from build123d import *

# Parameters (mm, degrees)
F0_R     = 3.175
F1_DEPTH = 3.048


with BuildPart() as f1:
    # F0 (on Front) → F1 (new body)
    with BuildSketch(Plane.XZ):
        with BuildLine():
            ThreePointArc((-23.2488528316, 63.9433400749), (-23.2457905964, 64.0827574545), (-23.2447697784, 64.222204724))
            ThreePointArc((-23.2447697784, 64.222204724), (-32.6010796562, 73.7457108348), (-42.2887946902, 64.5595320539))
            ThreePointArc((-42.2887946902, 64.5595320539), (-33.0778672203, 54.7021889169), (-23.2488528316, 63.9433400749))
        make_face()
        with Locations((-32.7697697784, 64.222204724)):
            Circle(F0_R, mode=Mode.SUBTRACT)
        with BuildLine():
            ThreePointArc((-23.2488528316, 63.9433400749), (-33.0778672203, 54.7021889169), (-42.2887946902, 64.5595320539))
            Line((-42.2887946902, 64.5595320539), (-48.5187123814, 15.4188098138))
            ThreePointArc((-48.5187123814, 15.4188098138), (-32.7820421912, 29.2971999803), (-17.023933011, 15.4431573445))
            Line((-17.023933011, 15.4431573445), (-23.2488528316, 63.9433400749))
        make_face()
        with Locations((-37.0385125279, 49.947404724)):
            Circle(F0_R, mode=Mode.SUBTRACT)
        with BuildLine():
            Line((-47.8670611639, 8.5143113042), (-48.5187123814, 15.4188098138))
            ThreePointArc((-48.5187123814, 15.4188098138), (-48.5745337038, 11.9305404647), (-47.8670611639, 8.5143113042))
        make_face()
        with BuildLine():
            ThreePointArc((-17.023933011, 15.4431573445), (-32.7820421912, 29.2971999803), (-48.5187123814, 15.4188098138))
            Line((-48.5187123814, 15.4188098138), (-47.8670611639, 8.5143113042))
            ThreePointArc((-47.8670611639, 8.5143113042), (-32.7807619476, -2.4527914704), (-17.6792895161, 8.4934086789))
            Line((-17.6792895161, 8.4934086789), (-17.023933011, 15.4431573445))
        make_face()
        with Locations((-32.7697697784, 13.422204724)):
            Circle(F0_R, mode=Mode.SUBTRACT)
        with BuildLine():
            ThreePointArc((-16.8947697784, 13.422204724), (-16.9270934943, 14.4347427029), (-17.023933011, 15.4431573445))
            Line((-17.023933011, 15.4431573445), (-17.6792895161, 8.4934086789))
            ThreePointArc((-17.6792895161, 8.4934086789), (-17.0921264739, 10.926783834), (-16.8947697784, 13.422204724))
        make_face()
        with BuildLine():
            ThreePointArc((-17.6792895161, 8.4934086789), (-32.7807619476, -2.4527914704), (-47.8670611639, 8.5143113042))
            Line((-47.8670611639, 8.5143113042), (-42.2526281336, -50.9727938316))
            ThreePointArc((-42.2526281336, -50.9727938316), (-33.2177648488, -40.5633365202), (-23.2447697784, -50.077795276))
            ThreePointArc((-23.2447697784, -50.077795276), (-25.8216856464, -56.5931426878), (-32.1581035098, -59.5831353213))
            Line((-32.1581035098, -59.5831353213), (16.7484584113, -58.0111983949))
            ThreePointArc((16.7484584113, -58.0111983949), (8.5569901399, -50.2053080097), (16.4934658536, -42.140295276))
            Line((16.4934658536, -42.140295276), (-13.7188447097, -42.140295276))
            ThreePointArc((-13.7188447097, -42.140295276), (-19.5984538444, -39.5413452668), (-21.6339307019, -33.4437081269))
            Line((-21.6339307019, -33.4437081269), (-17.6792895161, 8.4934086789))
        make_face()
        with BuildLine():
            ThreePointArc((-23.2447697784, -50.077795276), (-33.2177648488, -40.5633365202), (-42.2526281336, -50.9727938316))
            ThreePointArc((-42.2526281336, -50.9727938316), (-39.1807277317, -57.1223139339), (-32.7697697784, -59.602795276))
            Line((-32.7697697784, -59.602795276), (-32.1581035098, -59.5831353213))
            ThreePointArc((-32.1581035098, -59.5831353213), (-25.8216856464, -56.5931426878), (-23.2447697784, -50.077795276))
        make_face()
        with Locations((-32.7697697784, -50.077795276)):
            Circle(F0_R, mode=Mode.SUBTRACT)
        with BuildLine():
            Line((-32.1581035098, -59.5831353213), (-32.7697697784, -59.602795276))
            ThreePointArc((-32.7697697784, -59.602795276), (-32.4637787091, -59.5978790186), (-32.1581035098, -59.5831353213))
        make_face()
        with BuildLine():
            ThreePointArc((24.4309658536, -50.077795276), (22.1061259292, -44.4651352004), (16.4934658536, -42.140295276))
            ThreePointArc((16.4934658536, -42.140295276), (8.5569901399, -50.2053080097), (16.7484584113, -58.0111983949))
            ThreePointArc((16.7484584113, -58.0111983949), (22.195566768, -55.5995659532), (24.4309658536, -50.077795276))
        make_face()
        with Locations((16.4934658536, -50.077795276)):
            Circle(F0_R, mode=Mode.SUBTRACT)
    extrude(amount=F1_DEPTH)


solid = f1.part
Geometry: final body of the model. Coordinates: model frame, mm. A direction names the side the tool comes from. Round coordinates to 2 decimals unless told otherwise and drop trailing zeros. Loops run counter-clockwise (first coordinate to the right, second up) from the corner with the lowest first, then second, coordinate; pieces in that order, holes last.
Q1. Material intervals for L1, parallel to Z at x = -32.5, y = -2.3; L2, parallel to Z at x = 16.5, y = -0.3; L3, parallel to Z at x = -36, y = -1, sorted ascending.
Q2. Section B-B on z = -48.5. Return loops of the section in (x, y).
Q3. Section A-A on y = -1.65. State how many separate pieces and enclosed holes the cut face has, plus the area to 3 significant figures.
Q4. Section D-D on z = -5.5. Return loops of the section in (x, y), plus the area to 3 significant figures.
Q5. Pull-direction query (X, two-part tool) for faces 4 (the flat face through (-29, 0, -7)), 5 (the cylindrical face through (-35.94, -1.5, 13.56)), 6 (the flat face through (-45.1, -1.5, -20.8)), 7 (the cylindrical face through (-35.29, -1.5, -52.01)); classes: released by +X, released by -X, zero draft, split by the parting line, or undercut.
Q6. Pin query (flat end, axial travel): P1, Ø0.9, axis at x = -2.5, y = -2, coming from the +Z side. Return the tip coordinate at first contact, or that it passes through.
Q7. Section C-C on x = -15. Return loops of the section in (y, z).
Q8. Access query for faces 1 (the flat face through (2, -2, -42.14)), 2 (the flat face through (-45.36, -1.5, 40.33)), 3 (the flat face through (-19.684, -1.503, -12.769)). Directions: +Z, -Z, +X, -X, +Y, -Y. A direction counts if a zero-diameter tool reaches every point of the face in a straight line with its end or side. Return the directions, or none.
Evaluation:
1. L1: z = -59.6 to -53.24, -46.91 to 10.26, 16.59 to 61.06, 67.39 to 73.74
1. L2: z = -58.02 to -53.25, -46.9 to -42.14
1. L3: z = -59.04 to 46.95, 52.95 to 73.18
2. outline: (-42.49, -3.05) - (-35.52, -3.05) - (-35.52, 0) - (-42.49, 0) - close; (-30.01, -3.05) - (13.74, -3.05) - (13.74, 0) - (-30.01, 0) - close; (19.25, -3.05) - (24.27, -3.05) - (24.27, 0) - (19.25, 0) - close
3. separate pieces: 1
3. enclosed holes: 5
3. area: 3,810 mm2
4. outline: (-46.54, -3.05) - (-19, -3.05) - (-19, 0) - (-46.54, 0) - close
4. area: 84.0 mm2
5. face 4: zero draft
5. face 5: undercut
5. face 6: released by -X
5. face 7: undercut
6. P1: stops at z = -42.14
7. outline: (-3.05, -59.03) - (0, -59.03) - (0, -42.04) - (-3.05, -42.04) - close
8. face 1: +Z, +X, +Y, -Y
8. face 2: +Z, -X, +Y, -Y
8. face 3: +X, +Y, -Y
